```python
from build123d import *

# Parameters (mm, degrees)
BOSS_EXTRUDE1_DEPTH = 8
SKETCH2_W           = 16
SKETCH2_H           = 23.5
BOSS_EXTRUDE2_DEPTH = 3
SKETCH3_R           = 1.45
CUT_EXTRUDE1_DEPTH  = 3


with BuildPart() as part:
    # Sketch1 → Boss-Extrude1 (new body)
    with BuildSketch(Plane(origin=(0, 0, 0), x_dir=(1, 0, 0), z_dir=(0, 1, 0))):
        Polygon((-47.134549376, 16.069493776), (-47.134549376, 12.069493776), (-39.134549376, 7.069493776), (-31.134549376, 12.069493776), (-31.134549376, 16.069493776), (-39.134549376, 11.069493776), align=None)
    extrude(amount=BOSS_EXTRUDE1_DEPTH)

    # Sketch2 → Boss-Extrude2 (add)
    with BuildSketch(Plane(origin=(0, 8, 0), x_dir=(1, 0, 0), z_dir=(0, 1, 0))):
        with Locations((-39.134549376, 4.319493776)):
            Rectangle(SKETCH2_W, SKETCH2_H)
    extrude(amount=BOSS_EXTRUDE2_DEPTH)

    # Sketch3 → Cut-Extrude1 (cut)
    with BuildSketch(Plane(origin=(0, 11, 0), x_dir=(1, 0, 0), z_dir=(0, 1, 0))):
        with Locations(Location((-39.134549376, -2.430506224, 0), (0, 0, 270))):
            Circle(SKETCH3_R)
    extrude(amount=-CUT_EXTRUDE1_DEPTH, mode=Mode.SUBTRACT)


solid = part.part
```
Geometry check sheet. Reference: the model listing, model coordinates, mm. A direction names the side the tool comes from. Round coordinates to 2 decimals unless told otherwise and drop trailing zeros. Loops run counter-clockwise (first coordinate to the right, second up) from the corner with the lowest first, then second, coordinate; pieces in that order, holes last. Notation, with made-up numbers: (-32, -28.75) - (20, -28.75) arc R5 ccw to (20, -19.75) - close; hole circle Ø3 at (30.5, 27.25). An arc over 180 degrees is marked (long way). Use a Markdown table: item, result.
Q1. Draft check along Z on faces 1 (the flat face through (-39, 8, -2)), 2 (the flat face through (-39, 9, -16.069)), 3 (the flat face through (-39, 9, 7.431)), 4 (the cylindrical face through (-40.42, 9.52, 3.1)). Enter one of: released by +Z, released by -Z, zero draft, split by the parting line, or undercut.
Solutions:
| item | result |
|---|---|
| face 1 | zero draft |
| face 2 | released by -Z |
| face 3 | released by +Z |
| face 4 | undercut |
Q2. Access from +Z, -Z, +X, -X, +Y, -Y to the whole of each face (thin tool, end or side, straight path). Record for faces 5 (the flat face through (-39, 11, -4)), 6 (the flat face through (-39, 8, -14)), 7 (the flat face through (-35.191, 3.944, -9.534)), 8 (the flat face through (-43.191, 3.944, -9.604)).
Solutions:
| item | result |
|---|---|
| face 5 | +Z, -Z, +X, -X, +Y |
| face 6 | -Z, -Y |
| face 7 | +Z, +X, -Y |
| face 8 | +Z, -X, -Y |
Q3. Material ranges on line 1 (Y direction, x = -46, z = 6); line 2 (X direction, y = 3.25, z = -12.5); line 3 (Z direction, x = -37, y = 7.5), recorded low to high.
Solutions:
| item | result |
|---|---|
| line 1 | y = 8 to 11 |
| line 2 | x = -47.13 to -41.42, -36.85 to -31.13 |
| line 3 | z = -12.4 to -8.4 |
Q4. Cross-section at A-A on y = 9.25. Record the cut outline in (x, z).
Solutions:
| item | result |
|---|---|
| outline | (-47.13, -16.07) - (-31.13, -16.07) - (-31.13, 7.43) - (-47.13, 7.43) - close; hole circle Ø2.9 at (-39.13, 2.43) |
Q5. Cross-section at B-B on z = 2.5. Record the cut outline in (x, y).
Solutions:
| item | result |
|---|---|
| outline | (-47.13, 8) - (-40.58, 8) - (-40.58, 11) - (-47.13, 11) - close; (-37.69, 8) - (-31.13, 8) - (-31.13, 11) - (-37.69, 11) - close |
Q6. Go/stop test with flat-tipped pins: P1, Ø4, axis at x = -38, y = 3, coming from the -Z side; P2, Ø3, axis at x = -38, y = 4.5, coming from the +Z side. Record where each tip stops, or that it passes through.
Solutions:
| item | result |
|---|---|
| P1 | stops at z = -13.03 |
| P2 | stops at z = -7.07 |
Q7. Cross-section at D-D on x = -36.5. Record the cut outline in (y, z), plus the area to 4 significant figures.
Solutions:
| item | result |
|---|---|
| outline | (0, -12.72) - (8, -12.72) - (8, -16.07) - (11, -16.07) - (11, 7.43) - (8, 7.43) - (8, -8.72) - (0, -8.72) - close |
| area | 102.5 mm2 |
Q8. Cross-section at C-C on z = -9. Record the cut outline in (x, y).
Solutions:
| item | result |
|---|---|
| outline | (-47.13, 8) - (-42.22, 8) - (-42.22, 0) - (-36.05, 0) - (-36.05, 8) - (-31.13, 8) - (-31.13, 11) - (-47.13, 11) - close |
